Job drawing, mm, ordinate dimensions from the low corner. One solid piece. A direction names the side the tool comes from. Coordinates: 2 decimals unless noted, no trailing zeros. Write each loop counter-clockwise with the first axis right and the second up, starting at its lowest first coordinate (ties: lowest second). Pieces come first, ordered by that corner, then holes. Notation, with made-up numbers: (-27, 77.5) - (-9, 77.5) arc R21 ccw to (-9, 112.5) - close; hole circle Ø3 at (-20, 30). An arc over 180 degrees is marked (long way). Use one line per item in the form item = value. Start each with the question number.
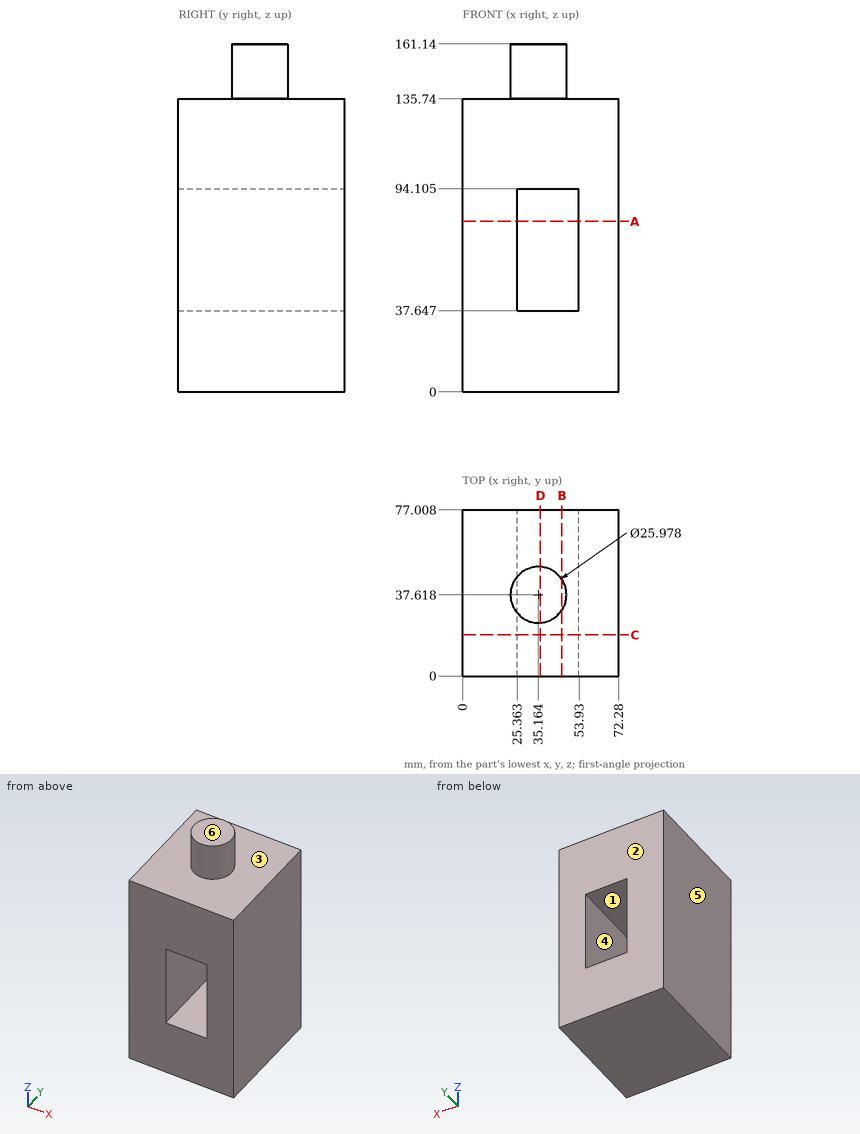
Q1. Drill centre lines: probe 1 along Z at (x, y) = (29, 41) (1 decimal); probe 2 along X at (y, z) = (47, 82); probe 3 along Z at (x, y) = (29, 59.5) (1 decimal). Where is each one in solid material? Low to high.
Q2. Pin check, flat tip, straight feed: P1, Ø10, axis at x = 12, y = 38, coming from the +Z side. Stop position of the tip, or through.
Q3. Mould opens along X. For the marked faces 4, 5 and 6 say: released by +X, released by -X, zero draft, split by the parting line, or undercut.
Q4. Which spindle directions (+Z, -Z, +X, -X, +Y, -Y) get a long thin tool onto all of the face, cutting with end or side? Do the marked faces 1, 2 and 3. Say none if no direction does.
Q5. Slice it at C-C (y = 19). List the corners of the cut face in (x, z) (1 decimal), plus the area to 3 significant figures.
Q6. Slice it at A-A (z = 79). List the corners of the cut face in (x, y), plus the area to 3 significant figures.
Q7. Slice it at B-B (x = 46). List the corners of the cut face in (y, z) (1 decimal).
Q8. Slice it at D-D (x = 36). List the corners of the cut face in (y, z) (1 decimal), plus the area to 3 significant figures.
Solution:
q1.probe_1 = 0 to 37.6, 94.1 to 161.1
q1.probe_2 = 0 to 25.36, 53.93 to 72.28
q1.probe_3 = 0 to 37.6, 94.1 to 135.7
q2.P1 = 135.74
q3.face_4 = undercut
q3.face_5 = released by -X
q3.face_6 = zero draft
q4.face_1 = +Y, -Y
q4.face_2 = +Z, -Z, +X, -X, +Y
q4.face_3 = +Z
q5.outline = (0, 0) - (72.3, 0) - (72.3, 135.7) - (0, 135.7) - close; hole (25.4, 37.6) - (53.9, 37.6) - (53.9, 94.1) - (25.4, 94.1) - close
q5.area = 8,200 mm2
q6.outline = (0, 0) - (25.36, 0) - (25.36, 77.01) - (0, 77.01) - close; (53.93, 0) - (72.28, 0) - (72.28, 77.01) - (53.93, 77.01) - close
q6.area = 3,370 mm2
q7.outline = (0, 0) - (77, 0) - (77, 37.6) - (0, 37.6) - close; (0, 94.1) - (77, 94.1) - (77, 135.7) - (44.8, 135.7) - (44.8, 161.1) - (30.5, 161.1) - (30.5, 135.7) - (0, 135.7) - close
q8.outline = (0, 0) - (77, 0) - (77, 37.6) - (0, 37.6) - close; (0, 94.1) - (77, 94.1) - (77, 135.7) - (50.6, 135.7) - (50.6, 161.1) - (24.7, 161.1) - (24.7, 135.7) - (0, 135.7) - close
q8.area = 6,760 mm2
